Autodesk Inventor part; units mm, degrees
ref_plane "Work Plane1" through (0, 700, 0) normal (0, 1, 0) x (-1, 0, 0)
ref_plane "YZ Plane" through (0, 0, 0) normal (1, 0, 0) x (0, 1, 0)
ref_plane "XY Plane" through (0, 0, 0) normal (0, 0, 1) x (1, 0, 0)
sketch "Sketch1" plane through (0, 0, 0) normal (0, 1, 0) x (-1, 0, 0)
  line L0 (0, -433.0127) -> (-375, -216.5064)
  line L1 (-375, -216.5064) -> (-375, 216.5064)
  line L2 (-375, 216.5064) -> (0, 433.0127)
  line L3 (0, 433.0127) -> (375, 216.5064)
  line L4 (375, 216.5064) -> (375, -216.5064)
  line L5 (375, -216.5064) -> (0, -433.0127)
  line L6 (0, -606.2178) -> (0, 606.2178)
  point P0 (0, 0)
  point P1 (0, 0)
  dimension "d0" = 750
ref_plane "Work Plane1" through (0, 700, 0) normal (0, 1, 0) x (-1, 0, 0)
sketch "Sketch2" plane through (0, 700, 0) normal (0, 1, 0) x (-1, 0, 0)
  line L0 (0, -392.5982) -> (-340, -196.2991)
  line L1 (-340, -196.2991) -> (-340, 196.2991)
  line L2 (-340, 196.2991) -> (0, 392.5982)
  line L3 (0, 392.5982) -> (340, 196.2991)
  line L4 (340, 196.2991) -> (340, -196.2991)
  line L5 (340, -196.2991) -> (0, -392.5982)
  point P0 (0, 0)
  point P1 (0, 0)
  dimension "d2" = 680
loft "Loft1" add profiles "Sketch1", "Sketch2"
sketch "Sketch3" plane through (340, 700, 196.2991) normal (0, 1, 0) x (1, 0, 0)
  circle A0 centre (-340, 196.2991) radius 255
  dimension "d7" = 510
extrude "Extrusion1" cut sketch "Sketch3" against normal blind 620
properties part number "smietnik1" material "Concrete"
For this review, take the finished solid that the model builds, in its own axes (mm). A direction names the side the tool comes from. Round coordinates to 2 decimals unless told otherwise and drop trailing zeros. Use one line per item in the form item = value.
1) Mouldability with a two-part tool opening along X and no side actions: class faces 1 (the face through (-5, 700, -256)), 2 (the face through (-55, 394, 249)) as pulls with the +X half, pulls with the -X half, needs draft (parallel to the pull), parting line crosses it, or undercut.
Solutions:
face_1 = needs draft
face_2 = undercut
2) Clearance check with flat-ended pins moving along their axes: P1, Ø8, axis at y = 311, z = -287, coming from the +X side; P2, Ø10, axis at x = 258, z = -138.5, coming from the -Y side; P3, Ø8, axis at x = -287, y = 71, coming from the -Z side; P4, Ø4, axis at y = 144.5, z = 220, coming from the +X side. State where each tip first meets the part, or that it passes through.
Solutions:
P1 = 228.74
P2 = 0
P3 = -265.53
P4 = 357.97
3) Wall thickness on probe 1 along Y at (x, z) = (11.5, 92.5); probe 2 along Z at (x, y) = (-121.5, 456); probe 3 along X at (y, z) = (517.5, 0) (3 decimals): over which ranges is each line inside the solid? List them lowest first.
Solutions:
probe_1 = 0 to 80
probe_2 = -336.54 to -224.19, 224.19 to 336.54
probe_3 = -349.125 to -255, 255 to 349.125
4) Tool access review of faces 3 (the face through (-5, 0, 6)), 4 (the face through (-4, 80, -4)): name each direction out of +Z, -Z, +X, -X, +Y, -Y from which nothing blocks a thin tool from reaching the whole face with its end or side.
Solutions:
face_3 = +Z, -Z, +X, -X, -Y
face_4 = +Y
